```python
from build123d import *

# Parameters (mm, degrees)
SKETCH_1_W           = 38.3
SKETCH_1_H           = 32
EXTRUDE_1_DEPTH      = 2
EXTRUDE_2_DEPTH      = 75
SKETCH_9_R           = 1.35
CUT_EXTRUDE_5_DEPTH  = 33
SKETCH_10_W          = 15.3
SKETCH_10_H          = 52
CUT_EXTRUDE_6_DEPTH  = 33
SKETCH_11_W          = 28.3
SKETCH_11_H          = 22
CUT_EXTRUDE_7_DEPTH  = 78
SKETCH_13_W          = 18
SKETCH_13_H          = 57
CUT_EXTRUDE_8_DEPTH  = 39.3
SKETCH_14_W          = 5
SKETCH_14_H          = 2
CUT_EXTRUDE_9_DEPTH  = 33
EXTRUDE_3_DEPTH      = 4
SKETCH_17_W          = 38.3
SKETCH_17_H          = 32
CUT_EXTRUDE_10_DEPTH = 57.2


with BuildPart() as part:
    # Эскиз1 → Бобышка-Вытянуть1 (new body)
    with BuildSketch(Plane(origin=(0, 0, 0), x_dir=(1, 0, 0), z_dir=(0, 1, 0))):
        Rectangle(SKETCH_1_W, SKETCH_1_H)
    extrude(amount=EXTRUDE_1_DEPTH)

    # Эскиз2 → Бобышка-Вытянуть2 (add)
    with BuildSketch(Plane(origin=(0, 2, 0), x_dir=(1, 0, 0), z_dir=(0, 1, 0))):
        Polygon((-19.15, 16), (19.15, 16), (19.15, -16), (-19.15, -16), (-19.15, -14), (17.15, -14), (17.15, 14), (-19.15, 14), align=None)
    extrude(amount=EXTRUDE_2_DEPTH)

    # Эскиз9 → Вырез-Вытянуть5 (cut, through all)
    with BuildSketch(Plane.XY.offset(16)):
        with Locations((-13.15, 69)):
            Circle(SKETCH_9_R)
        with Locations((-13.15, 10)):
            Circle(SKETCH_9_R)
    extrude(amount=-CUT_EXTRUDE_5_DEPTH, mode=Mode.SUBTRACT)

    # Эскиз10 → Вырез-Вытянуть6 (cut, through all)
    with BuildSketch(Plane.XY.offset(16)):
        with Locations((3.5, 36)):
            Rectangle(SKETCH_10_W, SKETCH_10_H)
    extrude(amount=-CUT_EXTRUDE_6_DEPTH, mode=Mode.SUBTRACT)

    # Эскиз11 → Вырез-Вытянуть7 (cut, through all)
    with BuildSketch(Plane.XZ):
        Rectangle(SKETCH_11_W, SKETCH_11_H)
    extrude(amount=-CUT_EXTRUDE_7_DEPTH, mode=Mode.SUBTRACT)

    # Эскиз13 → Вырез-Вытянуть8 (cut, through all)
    with BuildSketch(Plane(origin=(19.15, 0, 0), x_dir=(0, 0, -1), z_dir=(1, 0, 0))):
        with Locations((0, 38.5)):
            Rectangle(SKETCH_13_W, SKETCH_13_H)
    extrude(amount=-CUT_EXTRUDE_8_DEPTH, mode=Mode.SUBTRACT)

    # Эскиз14 → Вырез-Вытянуть9 (cut, through all)
    with BuildSketch(Plane(origin=(0, 0, -16), x_dir=(-1, 0, 0), z_dir=(0, 0, -1))):
        with Locations((-11.65, 71)):
            Rectangle(SKETCH_14_W, SKETCH_14_H)
        with Locations((1.65, 71)):
            Rectangle(SKETCH_14_W, SKETCH_14_H)
    extrude(amount=-CUT_EXTRUDE_9_DEPTH, mode=Mode.SUBTRACT)

    # Эскиз16 → Бобышка-Вытянуть3 (add)
    with BuildSketch(Plane.XY.offset(16)):
        Polygon((-19.15, 0), (-4.15, 0), (-4.15, 19.8), (-19.15, 19.8), (-19.15, 16.8), (-7.15, 16.8), (-7.15, 3.2), (-19.15, 3.2), align=None)
    extrude_3 = extrude(amount=EXTRUDE_3_DEPTH)

    # Зеркальное отражение1: Бобышка-Вытянуть3 across plane
    add(extrude_3.mirror(Plane.XY))

    # Эскиз17 → Вырез-Вытянуть10 (cut)
    with BuildSketch(Plane(origin=(0, 77, 0), x_dir=(1, 0, 0), z_dir=(0, 1, 0))):
        Rectangle(SKETCH_17_W, SKETCH_17_H)
    extrude(amount=-CUT_EXTRUDE_10_DEPTH, mode=Mode.SUBTRACT)


solid = part.part
```
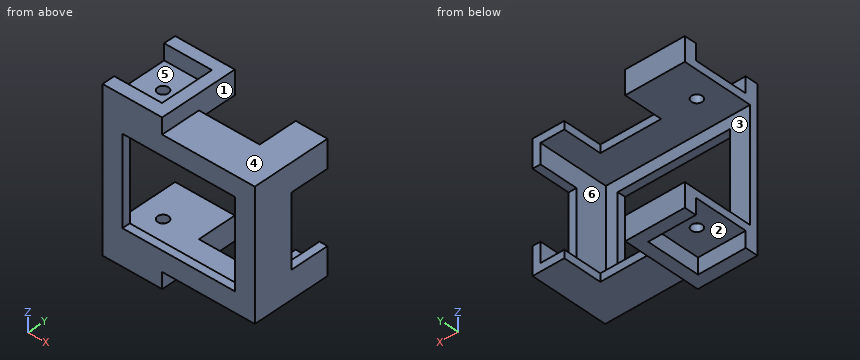
Geometry check sheet. Reference: the model listing, model coordinates, mm. Face numbers are marked on the shaded views. A direction names the side the tool comes from. Coordinates: 2 decimals unless noted, no trailing zeros. Loops run counter-clockwise (first coordinate to the right, second up) from the corner with the lowest first, then second, coordinate; pieces in that order, holes last. Notation, with made-up numbers: (82, 67.25) -> (131, 67.25) arc R34 ccw to (131, 99.25) -> close; hole circle Ø7 at (34.5, 37). An arc over 180 degrees is marked (long way). Put each result on its own line as item: value.
1) Tool access check on the marked faces 4, 5 and 6. Record the directions out of +Z, -Z, +X, -X, +Y, -Y that give a thin tool (end or side, any length) a straight path to the whole face; none if there is none.
Result set:
face 4: +Z, +X, +Y, -Y
face 5: +Z, -X
face 6: -X, +Y
2) Cross-section at D-D on x = -2. Record the boundary of the cut face in (y, z), plus the area to 3 significant figures.
Result set:
outline: (0, -16) -> (10, -16) -> (10, -14) -> (2, -14) -> (2, -11) -> (0, -11) -> close; (0, 11) -> (2, 11) -> (2, 14) -> (10, 14) -> (10, 16) -> (0, 16) -> close
area: 52.0 mm^2
3) Gauge pin test, flat ends, axial feed: pin 1 Ø1.5 at (x, y) = (13.5, 9.5) entering from +Z; pin 2 Ø1.8 at (y, z) = (9.5, 17.5) entering from +X; pin 3 Ø1 at (x, z) = (3.5, -15.5) entering from +Y; pin 4 Ø10 at (x, z) = (8.5, 4.5) entering from -Y. Record the tip position at first contact, or that the pin passes through.
Result set:
pin 1: stops at z = 16
pin 2: stops at x = -4.15
pin 3: stops at y = 10
pin 4: passes through
4) Cross-section at C-C on y = 9.5. Record the boundary of the cut face in (x, z), plus the area to 3 significant figures.
Result set:
outline: (-19.15, -16) -> (-14.4, -16) -> (-14.4, -14) -> (-19.15, -14) -> close; (-19.15, 14) -> (-14.4, 14) -> (-14.4, 16) -> (-19.15, 16) -> close; (-11.9, -16) -> (-7.15, -16) -> (-7.15, -20) -> (-4.15, -20) -> (-4.15, -16) -> (19.15, -16) -> (19.15, 16) -> (-4.15, 16) -> (-4.15, 20) -> (-7.15, 20) -> (-7.15, 16) -> (-11.9, 16) -> (-11.9, 14) -> (17.15, 14) -> (17.15, -14) -> (-11.9, -14) -> close
area: 223 mm^2
5) Release check for a two-part mould opening along Z. For the marked faces 1, 2 and 3 record: released by +Z, released by -Z, zero draft, split by the parting line, or undercut.
Result set:
face 1: zero draft
face 2: released by -Z
face 3: undercut
6) Cross-section at B-B on x = -13.15. Record the boundary of the cut face in (y, z), plus the area to 3 significant figures.
Result set:
outline: (0, -20) -> (3.2, -20) -> (3.2, -16) -> (8.65, -16) -> (8.65, -14) -> (2, -14) -> (2, -11) -> (0, -11) -> close; (0, 11) -> (2, 11) -> (2, 14) -> (8.65, 14) -> (8.65, 16) -> (3.2, 16) -> (3.2, 20) -> (0, 20) -> close; (11.35, -16) -> (16.8, -16) -> (16.8, -20) -> (19.8, -20) -> (19.8, -14) -> (11.35, -14) -> close; (11.35, 14) -> (19.8, 14) -> (19.8, 20) -> (16.8, 20) -> (16.8, 16) -> (11.35, 16) -> close
area: 130 mm^2
7) Cross-section at A-A on z = -0.5. Record the boundary of the cut face in (x, y).
Result set:
outline: (-19.15, 0) -> (-14.15, 0) -> (-14.15, 2) -> (-19.15, 2) -> close; (14.15, 0) -> (19.15, 0) -> (19.15, 10) -> (17.15, 10) -> (17.15, 2) -> (14.15, 2) -> close
8) Thickness scan on line 1 (Z direction, x = -10, y = 7.25); line 2 (Y direction, x = -13.15, z = 15.1); line 3 (Y direction, x = -10, z = -18). Record the ranges inside material, lowest first.
Result set:
line 1: z = -16 to -14, 14 to 16
line 2: y = 0 to 8.65, 11.35 to 19.8
line 3: y = 0 to 3.2, 16.8 to 19.8
